The listing builds one solid part. Answer for the finished solid, in the listing's coordinates (mm). A direction names the side the tool comes from. Give positions to 0.01 mm unless a question says otherwise; leave off trailing zeros. Loops run counter-clockwise (first coordinate to the right, second up) from the corner with the lowest first, then second, coordinate; pieces in that order, holes last. Notation, with made-up numbers: M 30,84 L 63,84 A27 cw 63,103 Z; hole C 22,9.25 d11. An arc over 180 degrees is marked long. Use one line per item in the form item = value. Start each with the question number.
1. The part is cut by section D-D (x = -12.5). Write down the section's boundary in (y, z) (1 decimal).
2. For faces 1 (the face through (-10, 35, 0)), 2 (the face through (-1.5, 28, 0)), 3 (the face through (19.625, 25, 0)), determine the directions among +Z, -Z, +X, -X, +Y, -Y from which every point of the face is accessible in a straight line to the end or side of a thin tool.
3. Each of these flat-tipped pins is pushed along its axis until it touches: pin 1 Ø1 at (x, z) = (-18.5, -1) entering from -Y; pin 2 Ø1 at (y, z) = (35.5, 0.5) entering from -X; pin 3 Ø1.5 at (y, z) = (22, -0.5) entering from -X; pin 4 Ø1 at (y, z) = (27.5, 0) entering from +X (3 decimals). Where does it stop, or does it pass through?
4. The part is cut by section B-B (x = 4.5). Write down the section's boundary in (y, z).
5. Straight lines are drawn through the part: line 1 (Y direction, x = -5, z = 1.2); line 2 (X direction, y = 28, z = -1.3); line 3 (Y direction, x = -11, z = -0.5) (3 decimals). For each, find the intervals that lie inside material, in ascending order. Write a range as from..to.
6. The part is cut by section C-C (y = 31.5). Write down the section's boundary in (x, z), and give its area (3 significant figures).
7. The part is cut by section A-A (z = 0.45). Write down the section's boundary in (x, y) (3 decimals), and give its area (3 significant figures).
8. The mould has two halves that part along X. Classify faces 4 (the face through (0, 11, 1.588)), 5 (the face through (-18.31, 30.98, 0.02)), 6 (the face through (-6, 24.2, 0)): released by +X, released by -X, zero draft, split by the parting line, or undercut.
from build123d import *

# Parameters (mm, degrees)
SKETCH1_W           = 39.69
SKETCH1_H           = 3.175
BOSS_EXTRUDE1_DEPTH = 12.7
CUT_EXTRUDE1_DEPTH  = 12.7
SKETCH4_W           = 6.35
SKETCH4_H           = 0.4
CUT_EXTRUDE2_DEPTH  = 12.7
BOSS_EXTRUDE2_DEPTH = 3.175
CUT_EXTRUDE3_DEPTH  = 3.175
BOSS_EXTRUDE3_DEPTH = 3.175
CUT_EXTRUDE4_DEPTH  = 3.175


with BuildPart() as part:
    # Sketch1 → Boss-Extrude1 (new body)
    with BuildSketch(Plane(origin=(0, 0, 0), x_dir=(1, 0, 0), z_dir=(0, 1, 0))):
        Rectangle(SKETCH1_W, SKETCH1_H)
    extrude(amount=BOSS_EXTRUDE1_DEPTH)

    # Sketch3 → Cut-Extrude1 (cut)
    with BuildSketch(Plane.XY.offset(1.5875)):
        with BuildLine():
            ThreePointArc((-10.653064207, 7.9375), (-10.188096222, 9.060032015), (-9.065564207, 9.525))
            Line((-9.065564207, 9.525), (-1.5875, 9.525))
            Line((-1.5875, 9.525), (-1.5875, 12.7))
            Line((-1.5875, 12.7), (-19.845, 12.7))
            Line((-19.845, 12.7), (-19.845, 1.599044979))
            Line((-19.845, 1.599044979), (-10.653064207, 6.35))
            Line((-10.653064207, 6.35), (-10.653064207, 7.9375))
        make_face()
        with BuildLine():
            Line((19.845, 12.7), (1.5875, 12.7))
            Line((1.5875, 12.7), (1.5875, 9.525))
            Line((1.5875, 9.525), (9.065564207, 9.525))
            ThreePointArc((9.065564207, 9.525), (10.188096222, 9.060032015), (10.653064207, 7.9375))
            Line((10.653064207, 7.9375), (10.653064207, 6.35))
            Line((10.653064207, 6.35), (19.845, 3.175))
            Line((19.845, 3.175), (19.845, 12.7))
        make_face()
    extrude(amount=-CUT_EXTRUDE1_DEPTH, mode=Mode.SUBTRACT)

    # Sketch4 → Cut-Extrude2 (cut)
    with BuildSketch(Plane.XY.offset(1.5875)):
        with Locations((0, 6.35)):
            Rectangle(SKETCH4_W, SKETCH4_H)
        Polygon((-0.2, 9.525), (0.2, 9.525), (0.2, 3.175), (0, 3.175), (-0.2, 3.175), align=None)
    extrude(amount=-CUT_EXTRUDE2_DEPTH, mode=Mode.SUBTRACT)

    # Sketch5 → Boss-Extrude2 (add)
    with BuildSketch(Plane.XY.offset(1.5875)):
        with BuildLine():
            Line((1.5875, 9.525), (9.065564207, 9.525))
            ThreePointArc((9.065564207, 9.525), (10.188096222, 9.060032015), (10.653064207, 7.9375))
            Line((10.653064207, 7.9375), (10.653064207, 6.35))
            Line((10.653064207, 6.35), (19.845, 3.175))
            Line((19.845, 3.175), (19.845, 0))
            Line((19.845, 0), (24.845, 0))
            Line((24.845, 0), (24.845, 37))
            Line((24.845, 37), (-24.845, 37))
            Line((-24.845, 37), (-24.845, 0))
            Line((-24.845, 0), (-19.845, 0))
            Line((-19.845, 0), (-19.845, 1.599044979))
            Line((-19.845, 1.599044979), (-10.653064207, 6.35))
            Line((-10.653064207, 6.35), (-10.653064207, 7.9375))
            ThreePointArc((-10.653064207, 7.9375), (-10.188096222, 9.060032015), (-9.065564207, 9.525))
            Line((-9.065564207, 9.525), (-1.5875, 9.525))
            Line((-1.5875, 9.525), (-1.5875, 12.7))
            Line((-1.5875, 12.7), (1.5875, 12.7))
            Line((1.5875, 12.7), (1.5875, 9.525))
        make_face()
    extrude(amount=-BOSS_EXTRUDE2_DEPTH)

    # Sketch6 → Cut-Extrude3 (cut)
    with BuildSketch(Plane.XY.offset(1.5875)):
        with BuildLine():
            Line((-10, 37), (-24.845, 37))
            Line((-24.845, 37), (-24.845, 27.75))
            Line((-24.845, 27.75), (-24.845, 18.5))
            Line((-24.845, 18.5), (-24.845, 9.25))
            Line((-24.845, 9.25), (-19.625, 23.125))
            Line((-19.625, 23.125), (-19.625, 27.75))
            ThreePointArc((-19.625, 27.75), (-18.270368863, 31.020368863), (-15, 32.375))
            Line((-15, 32.375), (-10, 32.375))
            Line((-10, 32.375), (-10, 37))
        make_face()
        with BuildLine():
            Line((24.845, 37), (10, 37))
            Line((10, 37), (10, 32.375))
            Line((10, 32.375), (15, 32.375))
            ThreePointArc((15, 32.375), (18.270368863, 31.020368863), (19.625, 27.75))
            Line((19.625, 27.75), (19.625, 23.125))
            Line((19.625, 23.125), (24.845, 9.25))
            Line((24.845, 9.25), (24.845, 18.5))
            Line((24.845, 18.5), (24.845, 37))
        make_face()
    extrude(amount=-CUT_EXTRUDE3_DEPTH, mode=Mode.SUBTRACT)

    # Sketch7 → Boss-Extrude3 (add)
    with BuildSketch(Plane.XY.offset(1.5875)):
        Polygon((0.2, 6.15), (0.2, 3.175), (-0.2, 3.175), (-0.2, 6.15), (-3.175, 6.15), (-3.175, 6.55), (-0.2, 6.55), (-0.2, 9.525), (0.2, 9.525), (0.2, 6.55), (3.175, 6.55), (3.175, 6.15), align=None)
    extrude(amount=-BOSS_EXTRUDE3_DEPTH)

    # Sketch8 → Cut-Extrude4 (cut)
    with BuildSketch(Plane.XY.offset(1.5875)):
        with BuildLine():
            Line((1.5, 24.2), (1.5, 32.586859967))
            ThreePointArc((1.5, 32.586859967), (0, 32.7), (-1.5, 32.586859967))
            Line((-1.5, 32.586859967), (-1.5, 24.2))
            Line((-1.5, 24.2), (-9.886859967, 24.2))
            ThreePointArc((-9.886859967, 24.2), (-10, 22.7), (-9.886859967, 21.2))
            Line((-9.886859967, 21.2), (-1.5, 21.2))
            Line((-1.5, 21.2), (-1.5, 12.813140033))
            ThreePointArc((-1.5, 12.813140033), (-0.752130419, 12.728325124), (0, 12.7))
            ThreePointArc((0, 12.7), (0.752130419, 12.728325124), (1.5, 12.813140033))
            Line((1.5, 12.813140033), (1.5, 21.2))
            Line((1.5, 21.2), (9.886859967, 21.2))
            ThreePointArc((9.886859967, 21.2), (9.971674876, 21.947869581), (10, 22.7))
            ThreePointArc((10, 22.7), (9.971674876, 23.452130419), (9.886859967, 24.2))
            Line((9.886859967, 24.2), (1.5, 24.2))
        make_face()
    extrude(amount=-CUT_EXTRUDE4_DEPTH, mode=Mode.SUBTRACT)


solid = part.part
Derived:
q1.outline = M 0,-1.6 L 32.4,-1.6 L 32.4,1.6 L 0,1.6 Z
q2.face_1 = +Z, -Z, -X, +Y
q2.face_2 = +Z, -Z
q2.face_3 = +Z, -Z, +X, +Y
q3.pin_1 = 0
q3.pin_2 = -10
q3.pin_3 = -20.33
q3.pin_4 = 19.625
q4.outline = M 0,-1.59 L 21.2,-1.59 L 21.2,1.59 L 0,1.59 Z; M 24.2,-1.59 L 37,-1.59 L 37,1.59 L 24.2,1.59 Z
q5.line_1 = 0..21.2, 24.2..37
q5.line_2 = -19.62..-1.5, 1.5..19.62
q5.line_3 = 0..32.375
q6.outline = M -17.71,-1.59 L -1.5,-1.59 L -1.5,1.59 L -17.71,1.59 Z; M 1.5,-1.59 L 17.71,-1.59 L 17.71,1.59 L 1.5,1.59 Z
q6.area = 103 mm2
q7.outline = M -24.845,0 L 24.845,0 L 24.845,9.25 L 19.625,23.125 L 19.625,27.75 A4.625 ccw 15,32.375 L 10,32.375 L 10,37 L -10,37 L -10,32.375 L -15,32.375 A4.625 ccw -19.625,27.75 L -19.625,23.125 L -24.845,9.25 Z; hole M -9.887,21.2 L -1.5,21.2 L -1.5,12.813 A10 ccw 1.5,12.813 L 1.5,21.2 L 9.887,21.2 A10 ccw 9.887,24.2 L 1.5,24.2 L 1.5,32.587 A10 ccw -1.5,32.587 L -1.5,24.2 L -9.887,24.2 A10 ccw Z
q7.area = 1,410 mm2
q8.face_4 = zero draft
q8.face_5 = released by -X
q8.face_6 = undercut
